Autodesk Inventor part; units mm, degrees
ref_plane "YZ Plane" through (0, 0, 0) normal (1, 0, 0) x (0, 1, 0)
ref_plane "XZ Plane" through (0, 0, 0) normal (0, 1, 0) x (-1, 0, 0)
ref_plane "XY Plane" through (0, 0, 0) normal (0, 0, 1) x (1, 0, 0)
sketch "Sketch1" plane through (0, 0, 0) normal (0, 0, 1) x (1, 0, 0)
  line L0 (3.4641, -6) -> (11.0268, -6)
  line L1 (11.0268, -2) -> (6.0268, -2)
  line L2 (6.0268, -2) -> (6.0268, 2)
  line L3 (6.0268, 2) -> (11.0268, 2)
  line L4 (11.0268, 6) -> (3.4641, 6)
  line L5 (16.0268, 2) -> (16.0268, 6)
  line L6 (16.0268, -6) -> (16.0268, -2)
  line L7 (16.0268, 6) -> (3.4641, 6)
  line L8 (3.4641, 6) -> (0, 0)
  line L9 (0, 0) -> (3.4641, -6)
  line L10 (3.4641, -6) -> (16.0268, -6)
  line L11 (16.0268, 2) -> (6.0268, 2)
  line L12 (6.0268, 2) -> (6.0268, -2)
  line L13 (6.0268, -2) -> (16.0268, -2)
  line L14 (16.0268, 6) -> (16.0268, 2)
  line L15 (16.0268, -2) -> (16.0268, -6)
  point P0 (0, 0)
  dimension "d8" = 10
  dimension "d9" = 10
extrude "Extrusion1" add sketch "Sketch1" along normal blind 10
chamfer "Chamfer2" distance 2 angle 45 4 edges at (16.0268, 4, 10) (16.0268, -4, 10) (16.0268, -4, 0) (16.0268, 4, 0)
sketch "Sketch3" plane through (3.4641, 6, 10) normal (0, 1, 0) x (1, 0, 0)
  line L0 (10.5627, 10) -> (0, 10)
  line L1 (12.5627, 8) -> (12.5627, 2)
  circle A0 centre (7.5627, 5) radius 0.75
  point P0 (-3.4641, 10)
  dimension "d13" = 1.5
  dimension "d14" = 5
  dimension "d15" = 5
extrude "Extrusion2" cut sketch "Sketch3" against normal blind 22.7
pattern_circular "Circular Pattern1" count 3 over 360 about axis through (0, 0, 0) along (0, 0, 1) of "Extrusion1", "Extrusion2", "Chamfer2"
sketch "Sketch4" plane through (0, 0, 10) normal (0, 0, 1) x (1, 0, 0)
  circle A0 centre (0, 0) radius 0.75
  dimension "d21" = 1.5
extrude "Extrusion3" cut sketch "Sketch4" against normal blind 8
sketch "Sketch6" plane through (0, 0, 0) normal (0, 0, -1) x (-1, 0, 0)
  line L0 (-1.5875, 1.5875) -> (1.5875, 1.5875)
  line L1 (1.5875, 1.5875) -> (1.5875, -1.5875)
  line L2 (1.5875, -1.5875) -> (-1.5875, -1.5875)
  line L3 (-1.5875, -1.5875) -> (-1.5875, 1.5875)
  point P0 (0, 0)
  dimension "d25" = 1.5875
  dimension "d26" = 3.175
  dimension "d27" = 3.175
  dimension "d28" = 1.5875
extrude "Extrusion4" cut sketch "Sketch6" against normal blind 11.1125
properties part number "Plunger2"
Input: part model. Units: mm. Frame: model coordinates. A direction names the side the tool comes from. Round coordinates to 2 decimals unless told otherwise and drop trailing zeros. Order: outer loops, then holes, each group sorted by start corner. A loop starts at its lowest first (then second) coordinate and runs counter-clockwise, first axis right, second up. Notation, with made-up numbers: (19.25, -8) - (60.25, -8) arc R36 ccw to (60.25, 31) - close; hole circle Ø8 at (50, -9). An arc over 180 degrees is marked (long way). Answer as a JSON object with one key per item and string values. Group by question number.
(1) Pin query (flat end, axial travel): P1, Ø1.6, axis at y = -0.5, z = 6, coming from the +X side; P2, Ø2.5, axis at x = 1, z = 4, coming from the +Y side; P3, Ø2.5, axis at x = 11.03, z = 5, coming from the +Y side. Return the tip coordinate at first contact, or that it passes through.
(2) Material intervals for probe 1 along X at (y, z) = (-7.5, 5.25); probe 2 along Y at (x, z) = (-5.25, 6); probe 3 along Y at (x, z) = (14.5, 3.5), sorted ascending. Write a range as from..to.
(3) Cut plane C-C (y = -3.5). Return loops of the section in (x, z), then the cut area to 3 significant figures.
(4) Draft query along Y for faces 1 (the face through (-6.725, -7.648, 4.93)), 2 (the face through (16.027, -4, 5)), 3 (the face through (10, -6, 5)). Return one class per face: released by +Y, released by -Y, zero draft, split by the parting line, or undercut.
(5) Reachability of faces 4 (the face through (-9.126, -7.863, 5.665)), 5 (the face through (10, 2, 5)), 6 (the face through (-1.588, 0, 5)) from +Z, -Z, +X, -X, +Y, -Y: full face, straight path, thin tool, end or side. Return the list, or none.
(6) Cut plane D-D (z = 1). Return loops of the section in (x, y), then the cut area to 3 significant figures.
(7) Cut plane A-A (x = 7.5). Return loops of the section in (y, z).
(8) Cut plane B-B (z = 6.25). Return loops of the section in (x, y), then the cut area to 3 significant figures.
Here are the results:
{
 "1": {"P1": "stops at x = 6.03", "P2": "stops at y = 12.43", "P3": "stops at y = 6"},
 "2": {"probe 1": "x = -11.26..-10.48, -7.65..-6.64, -2.02..2.6", "probe 2": "y = -15.48..-13.09, -5.09..5.09, 13.09..15.48", "probe 3": "y = -6..-2, 2..6"},
 "3": {"outline": "(-8.95, 0) - (14.03, 0) - (16.03, 2) - (16.03, 8) - (14.03, 10) - (-8.95, 10) - close; hole circle Ø1.5 at (11.03, 5)", "area": "244 mm^2"},
 "4": {"face 1": "undercut", "face 2": "zero draft", "face 3": "released by -Y"},
 "5": {"face 4": "none", "face 5": "+Z, -Z, +X", "face 6": "+Z, -Z"},
 "6": {"outline": "(-12.71, -10.01) - (-9.25, -12.01) - (-4.75, -4.22) - (-1.28, -6.22) - (-5.78, -14.01) - (-2.32, -16.01) - (3.46, -6) - (15.03, -6) - (15.03, -2) - (6.03, -2) - (6.03, 2) - (15.03, 2) - (15.03, 6) - (3.46, 6) - (-2.32, 16.01) - (-5.78, 14.01) - (-1.28, 6.22) - (-4.75, 4.22) - (-9.25, 12.01) - (-12.71, 10.01) - (-6.93, 0) - close; hole (-1.59, -1.59) - (1.59, -1.59) - (1.59, 1.59) - (-1.59, 1.59) - close", "area": "361 mm^2"},
 "7": {"outline": "(-6, 0) - (-2, 0) - (-2, 10) - (-6, 10) - close; (2, 0) - (6, 0) - (6, 10) - (2, 10) - close"},
 "8": {"outline": "(-13.21, -10.88) - (-9.75, -12.88) - (-4.75, -4.22) - (-1.28, -6.22) - (-6.28, -14.88) - (-2.82, -16.88) - (3.46, -6) - (16.03, -6) - (16.03, -2) - (6.03, -2) - (6.03, 2) - (16.03, 2) - (16.03, 6) - (3.46, 6) - (-2.82, 16.88) - (-6.28, 14.88) - (-1.28, 6.22) - (-4.75, 4.22) - (-9.75, 12.88) - (-13.21, 10.88) - (-6.93, 0) - close; hole (-1.59, -1.59) - (1.59, -1.59) - (1.59, 1.59) - (-1.59, 1.59) - close", "area": "385 mm^2"}
}
